Autodesk Inventor part; units mm, degrees
ref_plane "YZ Plane" through (0, 0, 0) normal (1, 0, 0) x (0, 1, 0)
ref_plane "XZ Plane" through (0, 0, 0) normal (0, 1, 0) x (-1, 0, 0)
ref_plane "XY Plane" through (0, 0, 0) normal (0, 0, 1) x (1, 0, 0)
sketch "Sketch1" plane through (0, 0, 0) normal (0, 1, 0) x (-1, 0, 0)
  circle A0 centre (0, 0) radius 12.7
  line L0 (34.29, 34.29) -> (-34.29, 34.29)
  line L1 (-34.29, 34.29) -> (-34.29, -34.29)
  line L2 (-34.29, -34.29) -> (34.29, -34.29)
  line L3 (34.29, -34.29) -> (34.29, 34.29)
  line L4 (34.29, 34.29) -> (-34.29, -34.29) construction
  line L5 (-34.29, 34.29) -> (34.29, -34.29) construction
  circle A1 centre (0, 0) radius 48.4934
  dimension "d0" = 25.4
  dimension "d4" = 68.58
  dimension "d5" = 68.58
extrude "Extrusion1" add sketch "Sketch1" along normal blind 2.54
sketch "Sketch2" plane through (0, 2.54, 0) normal (0, 1, 0) x (1, 0, 0)
  line L0 (-29.21, -29.21) -> (29.21, -29.21) construction
  line L1 (29.21, -29.21) -> (29.21, 29.21) construction
  line L2 (29.21, 29.21) -> (-29.21, 29.21) construction
  line L3 (-29.21, 29.21) -> (-29.21, -29.21) construction
  line L4 (-29.21, -29.21) -> (29.21, 29.21) construction
  line L5 (29.21, -29.21) -> (-29.21, 29.21) construction
  line L6 (34.29, 34.29) -> (-34.29, 34.29)
  line L7 (34.29, -34.29) -> (34.29, 34.29)
  circle A0 centre (0, 0) radius 41.3092 construction
  circle A1 centre (0, 0) radius 48.4934 construction
  dimension "d24" = 7.1842
hole "Hole1" at (-29.21, 2.54, -29.21) at (29.21, 2.54, -29.21) at (29.21, 2.54, 29.21) at (-29.21, 2.54, 29.21) direction (0, -1, 0) diameter 5.1054 end through all
sketch "Sketch3" plane through (0, 2.54, 0) normal (0, 1, 0) x (1, 0, 0)
  circle A0 centre (0, 0) radius 38.1
  circle A1 centre (0, 0) radius 12.7
  circle A2 centre (0, 0) radius 25.4
  circle A3 centre (0, 0) radius 47.7012
  dimension "d17" = 76.2
  dimension "d18" = 50.8
  dimension "d19" = 95.4024
sketch "Sketch4" plane through (0, 2.54, 0) normal (0, 1, 0) x (1, 0, 0)
  circle A0 centre (0, 0) radius 12.7
  circle A1 centre (0, 0) radius 45.72
  dimension "d20" = 91.44
extrude "Extrusion2" cut sketch "Sketch4" against normal blind 25.4 keep common part
properties part number "weldpart" material "Stainless Steel"
Could you check a few things on this model? Use its own coordinates, in mm. Give positions to 0.01 mm unless a question says otherwise; leave off trailing zeros. Loops run counter-clockwise (first coordinate to the right, second up) from the corner with the lowest first, then second, coordinate; pieces in that order, holes last. Notation, with made-up numbers: (-23.5, -33) -> (19.5, -33) arc R28 cw to (19.5, -4) -> close; hole circle Ø9 at (-29.75, 9). An arc over 180 degrees is marked (long way). Return JSON: item names as keys, results as strings.
Item 1: We'd pull the mould along Z, two halves only. Please class faces 1 (the cylindrical face through (31.475, 1.252, 30.388)), 2 (the flat face through (-10, 2.54, -10)), 3 (the cylindrical face through (43.61, 1.29, -13.73)): +Z half, -Z half, draft (parallel to the pull), parting line (faces both ways), or undercut.
Geometry results:
{"face 1": "undercut", "face 2": "draft", "face 3": "parting line"}
Item 2: If we section it at B-B on z = 0: List the corners of the cut face in (x, y) for me.
Geometry results:
{"outline": "(-45.72, 0) -> (-12.7, 0) -> (-12.7, 2.54) -> (-45.72, 2.54) -> close; (12.7, 0) -> (45.72, 0) -> (45.72, 2.54) -> (12.7, 2.54) -> close"}
Item 3: If we section it at D-D on z = -29.21: List the corners of the cut face in (x, y) for me.
Geometry results:
{"outline": "(-35.17, 0) -> (-31.76, 0) -> (-31.76, 2.54) -> (-35.17, 2.54) -> close; (-26.66, 0) -> (26.66, 0) -> (26.66, 2.54) -> (-26.66, 2.54) -> close; (31.76, 0) -> (35.17, 0) -> (35.17, 2.54) -> (31.76, 2.54) -> close"}
Item 4: I'm going to push flat-ended pins straight in: pin 1 (6.5 mm diameter, centred on x = 29.21, z = -29.21, fed in from +Y); pin 2 (4.5 mm diameter, centred on x = -29.21, z = 29.21, fed in from +Y); pin 3 (1 mm diameter, centred on y = 0.5, z = -8.5, fed in from +X); pin 4 (1 mm diameter, centred on x = -16, y = 1.5, fed in from +Z). Where does each tip first touch, or does it pass through?
Geometry results:
{"pin 1": "stops at y = 2.54", "pin 2": "passes through", "pin 3": "stops at x = 45.01", "pin 4": "stops at z = 43.01"}
Item 5: I need wall thicknesses on L1, parallel to X at y = 1.2, z = 29.21; L2, parallel to X at y = 0.5, z = -27. Which ranges of each line are inside material? Lowest first, please. Write a range as from..to.
Geometry results:
{"L1": "x = -35.17..-31.76, -26.66..26.66, 31.76..35.17", "L2": "x = -36.9..-30.49, -27.93..27.93, 30.49..36.9"}
Item 6: If we section it at C-C on y = 0.4: List the corners of the cut face in (x, z) for me.
Geometry results:
{"outline": "circle Ø91.44 at (0, 0); hole circle Ø5.11 at (-29.21, -29.21); hole circle Ø5.11 at (-29.21, 29.21); hole circle Ø25.4 at (0, 0); hole circle Ø5.11 at (29.21, -29.21); hole circle Ø5.11 at (29.21, 29.21)"}
Item 7: If we section it at A-A on x = 0: List the corners of the cut face in (y, z) for me.
Geometry results:
{"outline": "(0, -45.72) -> (2.54, -45.72) -> (2.54, -12.7) -> (0, -12.7) -> close; (0, 12.7) -> (2.54, 12.7) -> (2.54, 45.72) -> (0, 45.72) -> close"}
